Source: three-view drawing plus pictorial views. Frame: mm from the lowest corner of the part. Coordinates: 2 decimals unless noted, no trailing zeros. Loops run counter-clockwise (first coordinate to the right, second up) from the corner with the lowest first, then second, coordinate; pieces in that order, holes last. Notation, with made-up numbers: (87.5, 62) - (92.5, 62) arc R23 cw to (92.5, 100) - close; hole circle Ø8 at (45, 75.5). An arc over 180 degrees is marked (long way). Return JSON: item names as keys, results as strings.
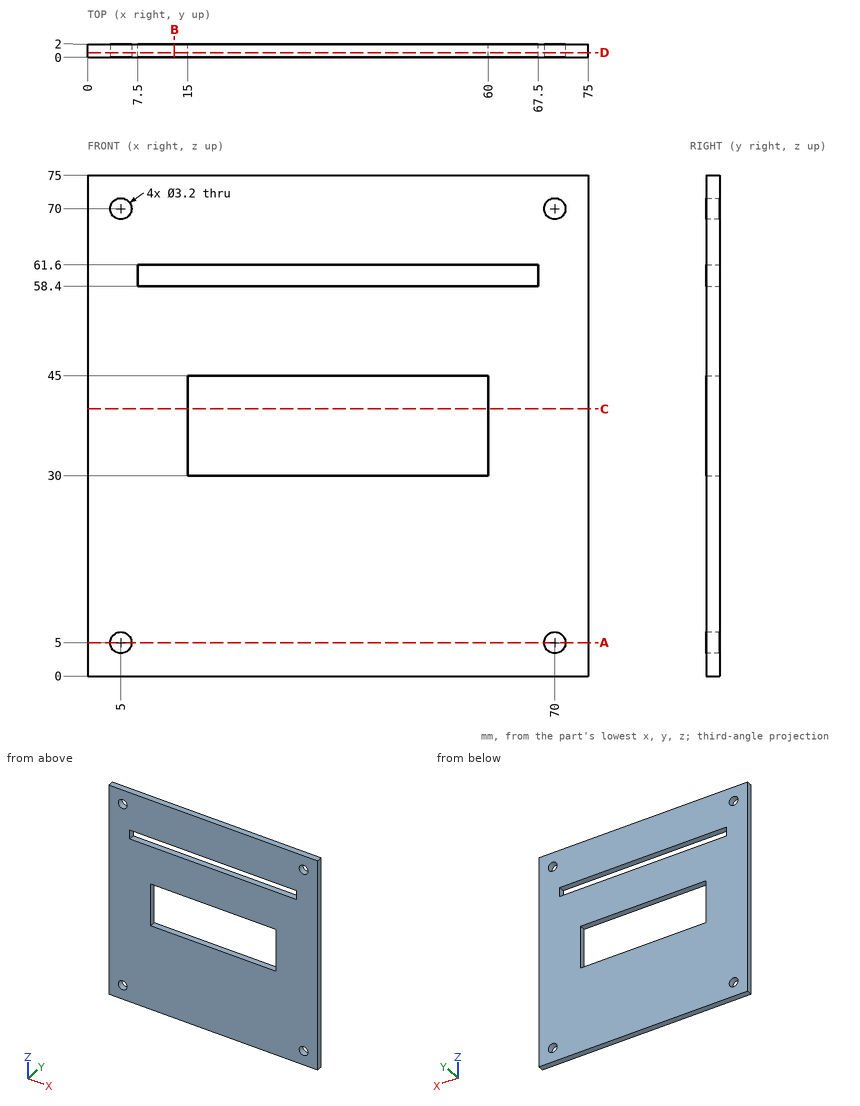
Item 1: Section query C-C, the plane z = 40. Return loops of the section in (x, y).
Worked out:
{"outline": "(0, 0) - (15, 0) - (15, 2) - (0, 2) - close; (60, 0) - (75, 0) - (75, 2) - (60, 2) - close"}
Item 2: Ray query, probe 1 along Z at (x, y) = (70, 1.35); probe 2 along Z at (x, y) = (55.5, 0.3). Return the intervals inside material, ascending. Write a range as from..to.
Worked out:
{"probe 1": "0..3.4, 6.6..68.4, 71.6..75", "probe 2": "0..30, 45..58.4, 61.6..75"}
Item 3: Section query D-D, the plane y = 0.7. Return loops of the section in (x, z), and give its area (3 significant figures).
Worked out:
{"outline": "(0, 0) - (75, 0) - (75, 75) - (0, 75) - close; hole circle Ø3.2 at (5, 5); hole circle Ø3.2 at (5, 70); hole (7.5, 58.4) - (67.5, 58.4) - (67.5, 61.6) - (7.5, 61.6) - close; hole (15, 30) - (60, 30) - (60, 45) - (15, 45) - close; hole circle Ø3.2 at (70, 5); hole circle Ø3.2 at (70, 70)", "area": "4,730 mm^2"}
Item 4: Section query A-A, the plane z = 5. Return loops of the section in (x, y).
Worked out:
{"outline": "(0, 0) - (3.4, 0) - (3.4, 2) - (0, 2) - close; (6.6, 0) - (68.4, 0) - (68.4, 2) - (6.6, 2) - close; (71.6, 0) - (75, 0) - (75, 2) - (71.6, 2) - close"}
Item 5: Section query B-B, the plane x = 13. Return loops of the section in (y, z).
Worked out:
{"outline": "(0, 0) - (2, 0) - (2, 58.4) - (0, 58.4) - close; (0, 61.6) - (2, 61.6) - (2, 75) - (0, 75) - close"}
